```python
from build123d import *

# Parameters (mm, degrees)
F1_DEPTH = 25.4
F0_R     = 12.7
F2_DEPTH = 50.8
F0_W     = 101.6
F0_H     = 12.7
F3_DEPTH = 63.5
F4_R     = 6.35
F5_DEPTH = 12.7


with BuildPart() as f1:
    # F0 (on Front) → F1 (new body)
    with BuildSketch(Plane.XZ):
        with BuildLine():
            ThreePointArc((25.4, 40.525289), (0, 15.125289), (-25.4, 40.525289))
            Line((-25.4, 40.525289), (-25.4, -22.974711))
            ThreePointArc((-25.4, -22.974711), (-32.839488, -40.935223), (-50.8, -48.374711))
            Line((-50.8, -48.374711), (50.8, -48.374711))
            ThreePointArc((50.8, -48.374711), (32.839488, -40.935223), (25.4, -22.974711))
            Line((25.4, -22.974711), (25.4, 40.525289))
        make_face()
    extrude(amount=F1_DEPTH)

    # F0 (on Front) → F2 (join)
    with BuildSketch(Plane.XZ):
        with BuildLine():
            ThreePointArc((25.4, 40.525289), (0, 65.925289), (-25.4, 40.525289))
            ThreePointArc((-25.4, 40.525289), (0, 15.125289), (25.4, 40.525289))
        make_face()
        with Locations((0, 40.525289)):
            Circle(F0_R, mode=Mode.SUBTRACT)
    extrude(amount=F2_DEPTH)

    # F0 (on Front) → F3 (join)
    with BuildSketch(Plane.XZ):
        with Locations((0, -54.724711)):
            Rectangle(F0_W, F0_H)
    extrude(amount=F3_DEPTH)

    # F4 (on face) → F5 (cut)
    with BuildSketch(Plane.XY.offset(-48.374711)):
        with Locations((-31.75, -44.45)):
            Circle(F4_R)
        with BuildLine():
            Line((-50.8, -63.5), (-38.1, -63.5))
            ThreePointArc((-38.1, -63.5), (-47.080256, -59.780256), (-50.8, -50.8))
            Line((-50.8, -50.8), (-50.8, -63.5))
        make_face()
        with BuildLine():
            ThreePointArc((50.8, -50.8), (47.080256, -59.780256), (38.1, -63.5))
            Line((38.1, -63.5), (50.8, -63.5))
            Line((50.8, -63.5), (50.8, -50.8))
        make_face()
        with Locations((31.75, -44.45)):
            Circle(F4_R)
    extrude(amount=-F5_DEPTH, mode=Mode.SUBTRACT)


solid = f1.part
```
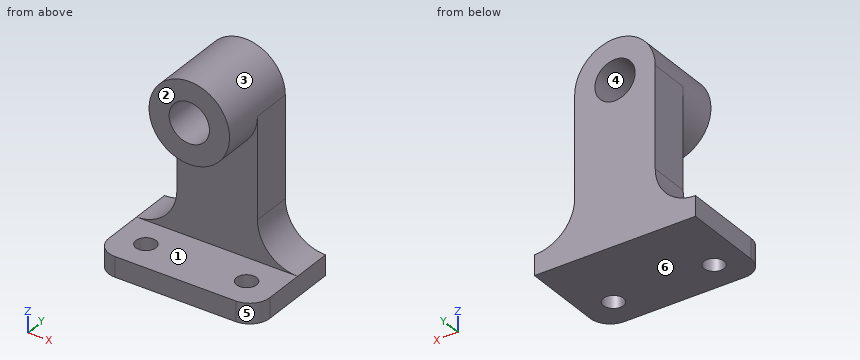
Source: CAD feature listing. Evaluate the final solid. Frame: model axes, mm. Face numbers are marked on the shaded views. A direction names the side the tool comes from. Round coordinates to 2 decimals unless told otherwise and drop trailing zeros. Write each loop counter-clockwise with the first axis right and the second up, starting at its lowest first coordinate (ties: lowest second). Pieces come first, ordered by that corner, then holes. Notation, with made-up numbers: M 81.25,31.5 L 111.25,31.5 A30 ccw 111.25,57.5 Z; hole C -24.5,16.25 d9. An arc over 180 degrees is marked long. Answer as a JSON object with one key per item and string values. Group by question number.
(1) Reachability of the marked faces 1, 2 and 3 from +Z, -Z, +X, -X, +Y, -Y: full face, straight path, thin tool, end or side. Return the list, or none.
(2) First-contact query: pin 1 (3 mm diameter, centred on x = 18.5, y = -37.5, fed in from +Z); pin 2 (19 mm diameter, centred on x = -1.5, y = -52, fed in from +Z); pin 3 (1.5 mm diameter, centred on y = -20, z = -37.5, fed in from +X). Flat tips, straight axial feed; report the tip coordinate or a pass-through.
(3) Mould query, pull axis X, two halves, no side actions, for the marked faces 4, 5 and 6. Classes: +X half, -X half, draft (parallel to the pull), parting line (faces both ways), or undercut.
(4) Section query A-A on y = -44.45. Output: boundary loops of the cut face in (x, z), then the cut area to 3 significant figures.
(5) Section query B-B on x = 0. Output: boundary loops of the cut face in (y, z).
(6) Ray query, line 1 (X direction, y = -44, z = -57); line 2 (Z direction, x = 0, y = -32); line 3 (Z direction, x = 3.5, y = -15). Return the intervals inside material, ascending. Write a range as [from, to].
(7) Section query D-D on y = -17.5. Output: boundary loops of the cut face in (x, z).
(8) Section query C-C on y = -30.5. Output: boundary loops of the cut face in (x, z), then the cut area to 3 significant figures.
Computed values:
{
 "1": {"face 1": "+X, -X, -Y", "face 2": "+Z, +X, -X, -Y", "face 3": "-Y"},
 "2": {"pin 1": "z = 59.4", "pin 2": "z = 65.93", "pin 3": "x = 30.51"},
 "3": {"face 4": "undercut", "face 5": "+X half", "face 6": "draft"},
 "4": {"outline": "M -50.8,-61.07 L -38.1,-61.07 L -38.1,-48.37 L -50.8,-48.37 Z; M -25.4,-61.07 L 25.4,-61.07 L 25.4,-48.37 L -25.4,-48.37 Z; C 0,40.53 d50.8; M 38.1,-61.07 L 50.8,-61.07 L 50.8,-48.37 L 38.1,-48.37 Z; hole C 0,40.53 d25.4", "area": "2,490 mm^2"},
 "5": {"outline": "M -63.5,-61.07 L 0,-61.07 L 0,27.83 L -50.8,27.83 L -50.8,15.13 L -25.4,15.13 L -25.4,-48.37 L -63.5,-48.37 Z; M -50.8,53.23 L 0,53.23 L 0,65.93 L -50.8,65.93 Z"},
 "6": {"line 1": "[-50.8, -38.08], [-25.42, 25.42], [38.08, 50.8]", "line 2": "[-61.07, -48.37], [15.13, 27.83], [53.23, 65.93]", "line 3": "[-61.07, 28.32], [52.73, 65.68]"},
 "7": {"outline": "M -50.8,-61.07 L 50.8,-61.07 L 50.8,-48.37 A25.4 cw 25.4,-22.97 L 25.4,40.53 A25.4 ccw -25.4,40.53 L -25.4,-22.97 A25.4 cw -50.8,-48.37 Z; hole C 0,40.53 d25.4"},
 "8": {"outline": "M -50.8,-61.07 L 50.8,-61.07 L 50.8,-48.37 L -50.8,-48.37 Z; C 0,40.53 d50.8; hole C 0,40.53 d25.4", "area": "2,810 mm^2"}
}
